```python
from build123d import *

# Parameters (mm, degrees)
BOX046_W          = 13
BOX046_H          = 0.4
BOX046_DEPTH      = 0.7
BOX045_W          = 13
BOX045_H          = 0.4
BOX045_DEPTH      = 1.3
BOX044_W          = 1
BOX044_H          = 14
BOX044_DEPTH      = 0.9
BOX043_W          = 1
BOX043_H          = 14
BOX043_DEPTH      = 0.9
BOX042_W          = 0.5
BOX042_H          = 14
BOX042_DEPTH      = 1.3
BOX041_W          = 0.5
BOX041_H          = 14
BOX041_DEPTH      = 1.3
BOX040_W          = 14
BOX040_H          = 14
BOX040_DEPTH      = 0.3
CYLINDER011_R     = 0.6
CYLINDER011_DEPTH = 0.6
CYLINDER012_R     = 0.6
CYLINDER012_DEPTH = 0.6
BOX055_W          = 8
BOX055_H          = 8.6
BOX055_DEPTH      = 2.1
BOX047_W          = 5
BOX047_H          = 4
BOX047_DEPTH      = 0.7


with BuildPart() as obj1:
    # Box046 → Box046 (new body)
    with BuildSketch(Plane(origin=(-6.5, -7, 0.3), x_dir=(1, 0, 0), z_dir=(0, 0, 1))):
        with Locations((6.5, 0.2)):
            Rectangle(BOX046_W, BOX046_H)
    extrude(amount=BOX046_DEPTH)


with BuildPart() as obj2:
    # Box045 → Box045 (new body)
    with BuildSketch(Plane(origin=(-6.5, 6.6, 0.3), x_dir=(1, 0, 0), z_dir=(0, 0, 1))):
        with Locations((6.5, 0.2)):
            Rectangle(BOX045_W, BOX045_H)
    extrude(amount=BOX045_DEPTH)


with BuildPart() as obj3:
    # Box044 → Box044 (new body)
    with BuildSketch(Plane(origin=(6.5, -7, 1.6), x_dir=(1, 0, 0), z_dir=(0, 0, 1))):
        with Locations((0.5, 7)):
            Rectangle(BOX044_W, BOX044_H)
    extrude(amount=BOX044_DEPTH)


with BuildPart() as obj4:
    # Box043 → Box043 (new body)
    with BuildSketch(Plane(origin=(-7.5, -7, 1.6), x_dir=(1, 0, 0), z_dir=(0, 0, 1))):
        with Locations((0.5, 7)):
            Rectangle(BOX043_W, BOX043_H)
    extrude(amount=BOX043_DEPTH)


with BuildPart() as obj5:
    # Box042 → Box042 (new body)
    with BuildSketch(Plane(origin=(6.5, -7, 0.3), x_dir=(1, 0, 0), z_dir=(0, 0, 1))):
        with Locations((0.25, 7)):
            Rectangle(BOX042_W, BOX042_H)
    extrude(amount=BOX042_DEPTH)


with BuildPart() as obj6:
    # Box041 → Box041 (new body)
    with BuildSketch(Plane(origin=(-7, -7, 0.3), x_dir=(1, 0, 0), z_dir=(0, 0, 1))):
        with Locations((0.25, 7)):
            Rectangle(BOX041_W, BOX041_H)
    extrude(amount=BOX041_DEPTH)


with BuildPart() as obj7:
    # Box040 → Box040 (new body)
    with BuildSketch(Plane(origin=(-7, -7, 0), x_dir=(1, 0, 0), z_dir=(0, 0, 1))):
        with Locations((7, 7)):
            Rectangle(BOX040_W, BOX040_H)
    extrude(amount=BOX040_DEPTH)


with BuildPart() as obj8:
    # Cylinder011 → Cylinder011 (new body)
    with BuildSketch(Plane(origin=(-5.5, -5.5, -0.6), x_dir=(1, 0, 0), z_dir=(0, 0, 1))):
        Circle(CYLINDER011_R)
    extrude(amount=CYLINDER011_DEPTH)


with BuildPart() as obj9:
    # Cylinder012 → Cylinder012 (new body)
    with BuildSketch(Plane(origin=(5.5, 5.5, -0.6), x_dir=(1, 0, 0), z_dir=(0, 0, 1))):
        Circle(CYLINDER012_R)
    extrude(amount=CYLINDER012_DEPTH)


with BuildPart() as obj10:
    # Box055 → Box055 (new body)
    with BuildSketch(Plane(origin=(-4, -5.6, 0.3), x_dir=(1, 0, 0), z_dir=(0, 0, 1))):
        with Locations((4, 4.3)):
            Rectangle(BOX055_W, BOX055_H)
    extrude(amount=BOX055_DEPTH)


with BuildPart() as obj11:
    # Box047 → Box047 (new body)
    with BuildSketch(Plane(origin=(-2.5, -1, -0.7), x_dir=(1, 0, 0), z_dir=(0, 0, 1))):
        with Locations((2.5, 2)):
            Rectangle(BOX047_W, BOX047_H)
    extrude(amount=BOX047_DEPTH)

    # Fusion011: union obj1, obj2, obj3, obj4, obj5, obj6, obj7, obj8, obj9, obj10
    add(obj1.part)
    add(obj2.part)
    add(obj3.part)
    add(obj4.part)
    add(obj5.part)
    add(obj6.part)
    add(obj7.part)
    add(obj8.part)
    add(obj9.part)
    add(obj10.part)


solid = obj11.part
```
Check sheet for the modelled part. Datum: model origin and axes. Units: mm. A direction names the side the tool comes from. Round coordinates to 2 decimals unless told otherwise and drop trailing zeros. Order: outer loops, then holes, each group sorted by start corner. A loop starts at its lowest first (then second) coordinate and runs counter-clockwise, first axis right, second up.
1) Section check B-B (y = 3.75). Record the boundary of the cut face in (x, z).
2) Go/stop test with flat-tipped pins: pin 1 Ø1.5 at (x, y) = (3.5, 3.5) entering from -Z; pin 2 Ø1.1 at (y, z) = (2, 1.5) entering from +X; pin 3 Ø4 at (x, y) = (-1, -1) entering from +Z; pin 4 Ø1 at (x, z) = (3, 2) entering from -Y. Record where each tip stops, or that it passes through.
3) Mould release check, pull along X, two halves, no side actions. Record for faces 6 (the flat face through (-7.5, 0, 2)), 7 (the flat face through (-0.1, -1.5, 0)), 8 (the flat face through (0, 4, 0.3)): +X half, -X half, draft (parallel to the pull), parting line (faces both ways), or undercut.
4) Section check D-D (z = 2). Record the boundary of the cut face in (x, y).
5) Tool access check on faces 1 (the flat face through (-7, 0, 1)), 2 (the flat face through (-7, 0, 2.5)), 3 (the flat face through (6.5, 0, 1)), 4 (the flat face through (0, 1, -0.7)), 5 (the cylindrical face through (5.78, 4.97, -0.3)). Record the directions out of +Z, -Z, +X, -X, +Y, -Y that give a thin tool (end or side, any length) a straight path to the whole face; none if there is none.
6) Section check C-C (x = 0). Record the boundary of the cut face in (y, z).
7) Scan lines: line 1 (Y direction, x = -3.25, z = 0.6); line 2 (X direction, y = -5.5, z = 1.8); line 3 (X direction, y = -1.5, z = 0.55). Record each from-to range of solid material in increasing order.
8) Section check A-A (z = -0.25). Record the boundary of the cut face in (x, y), and give its area (3 significant figures).
Result:
1. outline: (-7.5, 1.6) - (-7, 1.6) - (-7, 0) - (7, 0) - (7, 1.6) - (7.5, 1.6) - (7.5, 2.5) - (6.5, 2.5) - (6.5, 0.3) - (-6.5, 0.3) - (-6.5, 2.5) - (-7.5, 2.5) - close
2. pin 1: stops at z = 0
2. pin 2: stops at x = 7.5
2. pin 3: stops at z = 2.4
2. pin 4: stops at y = -5.6
3. face 6: -X half
3. face 7: draft
3. face 8: undercut
4. outline: (-7.5, -7) - (-6.5, -7) - (-6.5, 7) - (-7.5, 7) - close; (-4, -5.6) - (4, -5.6) - (4, 3) - (-4, 3) - close; (6.5, -7) - (7.5, -7) - (7.5, 7) - (6.5, 7) - close
5. face 1: -Z, -X, +Y, -Y
5. face 2: +Z, +X, -X, +Y, -Y
5. face 3: +Z
5. face 4: -Z, +X, -X, +Y, -Y
5. face 5: -Z
6. outline: (-7, 0) - (-1, 0) - (-1, -0.7) - (3, -0.7) - (3, 0) - (7, 0) - (7, 1.6) - (6.6, 1.6) - (6.6, 0.3) - (3, 0.3) - (3, 2.4) - (-5.6, 2.4) - (-5.6, 0.3) - (-6.6, 0.3) - (-6.6, 1) - (-7, 1) - close
7. line 1: y = -7 to -6.6, -5.6 to 3, 6.6 to 7
7. line 2: x = -7.5 to -6.5, -4 to 4, 6.5 to 7.5
7. line 3: x = -7 to -6.5, -4 to 4, 6.5 to 7
8. outline: circle Ø1.2 at (-5.5, -5.5); (-2.5, -1) - (2.5, -1) - (2.5, 3) - (-2.5, 3) - close; circle Ø1.2 at (5.5, 5.5)
8. area: 22.3 mm2
